```python
from build123d import *


with BuildPart() as part:
    # Эскиз1 → Повернуть1 (revolve)
    with BuildSketch(Plane.XY):
        with BuildLine():
            Line((-88.367595483, 25.597236847), (-88.367595483, 36.95))
            Line((-88.367595483, 36.95), (-87.867595483, 37.45))
            Line((-87.867595483, 37.45), (-48.067595483, 37.45))
            ThreePointArc((-48.067595483, 37.45), (-44.532061577, 38.914466094), (-43.067595483, 42.45))
            Line((-43.067595483, 42.45), (-43.067595483, 68.6))
            Line((-43.067595483, 68.6), (-35.767595483, 68.6))
            Line((-35.767595483, 68.6), (-35.767595483, 95.25))
            Line((-35.767595483, 95.25), (-25.917595483, 105.1))
            Line((-25.917595483, 105.1), (-20.767595483, 105.1))
            Line((-20.767595483, 105.1), (-20.767595483, 124.82))
            Line((-20.767595483, 124.82), (-10.567595483, 124.82))
            Line((-10.567595483, 124.82), (-10.567595483, 94.97))
            Line((-10.567595483, 94.97), (-7.467595483, 94.97))
            Line((-7.467595483, 94.97), (-7.467595483, 90.15))
            Line((-7.467595483, 90.15), (-22.667595483, 90.15))
            Line((-22.667595483, 90.15), (-22.667595483, 67.2))
            Line((-22.667595483, 67.2), (-23.667595483, 66.2))
            Line((-23.667595483, 66.2), (-26.227595483, 66.2))
            Line((-26.227595483, 66.2), (-26.227595483, 47.99))
            Line((-26.227595483, 47.99), (-33.667595483, 35.103541992))
            Line((-33.667595483, 35.103541992), (-33.667595483, 20.76))
            Line((-33.667595483, 20.76), (-86.870219917, 23.911307188))
            Line((-86.870219917, 23.911307188), (-88.367595483, 25.597236847))
        make_face()
    revolve(axis=Axis((0, 0, 0), (-1, 0, 0)))


solid = part.part
```
The listing builds one solid part. Answer for the finished solid, in the listing's coordinates (mm). A direction names the side the tool comes from. Round coordinates to 2 decimals unless told otherwise and drop trailing zeros. Loops run counter-clockwise (first coordinate to the right, second up) from the corner with the lowest first, then second, coordinate; pieces in that order, holes last. Notation, with made-up numbers: (23, 71.25) - (38, 71.25) arc R22 cw to (38, 89.25) - close; hole circle Ø4 at (-40, -22.5). An arc over 180 degrees is marked (long way). Return JSON: item names as keys, results as strings. Group by question number.
1. The mould has two halves that part along Z. Classify faces 1 (the cylindrical face through (-67.689, 34.594, 14.344)), 2 (the flat face through (-88.368, -8, -25)), 3 (the conical face through (-60.641, -4.847, 21.826)): pulls with the +Z half, pulls with the -Z half, needs draft (parallel to the pull), parting line crosses it, or undercut.
2. Consider probe 1 along Z at (x, y) = (-24.2, 0); probe 2 along Y at (x, z) = (-13, 0). Determine where each line is inside the solid, lowest interval first.
3. The part is cut by section A-A on x = -39. Determine the outline of the cut face in (y, z), then the cut area to 3 significant figures.
4. Each of these flat-tipped pins is pushed along its axis until it touches: P1, Ø1.5, axis at y = 16.5, z = -30.5, coming from the +X side; P2, Ø6, axis at x = -16.5, z = 19, coming from the -Y side; P3, Ø8, axis at x = -22, z = 34, coming from the +Y side. Where does it stop, or does it pass through?
5. Which of the six approach directions +Z, -Z, +X, -X, +Y, -Y give full straight-line access (tool end or side, diameter ignored) to faces 4 (the cylindrical face through (-39.37, 65.43, -20.61)), 5 (the flat face through (-33.668, 15, 15)), 6 (the cylindrical face through (-15.596, 57.597, 110.737))?
Resolved:
{
 "1": {"face 1": "parting line crosses it", "face 2": "needs draft", "face 3": "undercut"},
 "2": {"probe 1": "z = -105.1 to -66.2, 66.2 to 105.1", "probe 2": "y = -124.82 to -90.15, 90.15 to 124.82"},
 "3": {"outline": "circle Ø137.2 at (0, 0); hole circle Ø42.15 at (0, 0)", "area": "13,400 mm²"},
 "4": {"P1": "stops at x = -33.48", "P2": "stops at y = -123.79", "P3": "stops at y = 121.11"},
 "5": {"face 4": "-X", "face 5": "+X", "face 6": "+X, -X"}
}
